Read the model definition and answer for the solid it produces. Units are mm, in the model's axes. Face numbers are marked on the shaded views. A direction names the side the tool comes from. Coordinates: 2 decimals unless noted, no trailing zeros. Write each loop counter-clockwise with the first axis right and the second up, starting at its lowest first coordinate (ties: lowest second). Pieces come first, ordered by that corner, then holes. Notation, with made-up numbers: (64.5, -7) - (75.5, -7) arc R7 cw to (75.5, 6) - close; hole circle Ø4 at (7, 20). An arc over 180 degrees is marked (long way). Return JSON: item names as keys, results as strings.
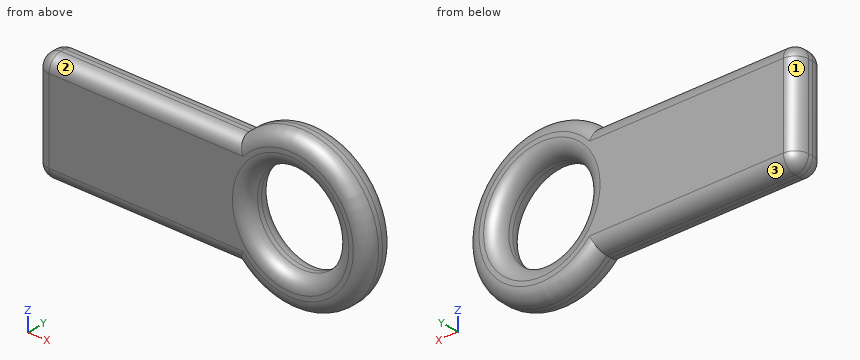
```python
from build123d import *

# Parameters (mm, degrees)
SKETCH1_R      = 50
EXTRUDE1_DEPTH = 35
FILLET1_R      = 15
FILLET2_R      = 15


with BuildPart() as part:
    # Sketch1 → Extrude1 (new body)
    with BuildSketch(Plane(origin=(0, 0, 0), x_dir=(1, 0, 0), z_dir=(0, 1, 0))):
        with BuildLine():
            Line((0, 0), (225.000255868, 0))
            ThreePointArc((225.000255868, 0), (369.65, 60.555), (225.000255868, 121.11))
            Line((225.000255868, 121.11), (0, 121.11))
            Line((0, 121.11), (0, 0))
        make_face()
        with Locations(Location((284.65, 60.555, 0), (0, 0, 270))):
            Circle(SKETCH1_R, mode=Mode.SUBTRACT)
    extrude(amount=EXTRUDE1_DEPTH)

    # Fillet1
    fillet1_edges = [part.edges().sort_by_distance(p)[0] for p in [
        (369.65, 35, -60.555),
        (284.65, 0, -110.555),
        (284.65, 35, -110.555),
        (112.500127934, 35, -121.11),
        (112.500127934, 0, -121.11),
        (369.65, 0, -60.555),
        (112.500127934, 0, 0),
        (112.500127934, 35, 0),
    ]]
    fillet(fillet1_edges, radius=FILLET1_R)

    # Fillet2
    fillet2_edges = [part.edges().sort_by_distance(p)[0] for p in [
        (0, 17.5, -121.11),
        (0, 0, -60.555),
        (0, 17.5, 0),
        (0, 35, -60.555),
        (0, 30.606601718, -4.393398282),
        (0, 4.393398282, -4.393398282),
        (0, 30.606601718, -116.716601718),
        (0, 4.393398282, -116.716601718),
    ]]
    fillet(fillet2_edges, radius=FILLET2_R)


solid = part.part
```
(1) A cutting plane is placed at A-A (x = 191.5). Determine the outline of the cut face in (y, z).
Answer:
{"outline": "(0, -106.11) arc R15 ccw to (15, -121.11) - (20, -121.11) arc R15 ccw to (35, -106.11) - (35, -15) arc R15 ccw to (20, 0) - (15, 0) arc R15 ccw to (0, -15) - close"}
(2) Which of the six approach directions +Z, -Z, +X, -X, +Y, -Y give full straight-line access (tool end or side, diameter ignored) to the marked faces 1, 2 and 3?
Answer:
{"face 1": "+Z, -Z, -X, +Y", "face 2": "+Z, -X, -Y", "face 3": "-Z, -X, +Y"}
(3) Flat-ended cylindrical pins translate along their axes: P1, Ø4, axis at y = 15.5, z = -90.5, coming from the +X side (3 decimals); P2, Ø10, axis at y = 28, z = -78, coming from the -X side; P3, Ø5, axis at x = 60, y = 20, coming from the +Z side; P4, Ø12, axis at y = 9, z = -89.5, coming from the -X side. Find the tip coordinate at first contact, or state that the pin passes through.
Answer:
{"P1": "x = 364.925", "P2": "x = 0.3", "P3": "z = 0", "P4": "x = 0"}
(4) Straight lines are drawn through the part: line 1 (Z direction, x = 184.5, y = 18); line 2 (X direction, y = 4, z = -69.5); line 3 (X direction, y = 3, z = -67.5). For each, find the intervals that lie inside material, in ascending order. Write a range as from..to.
Answer:
{"line 1": "-121.11..0", "line 2": "4.8..230.58, 338.72..364.35", "line 3": "6..229.08, 340.22..363.34"}
